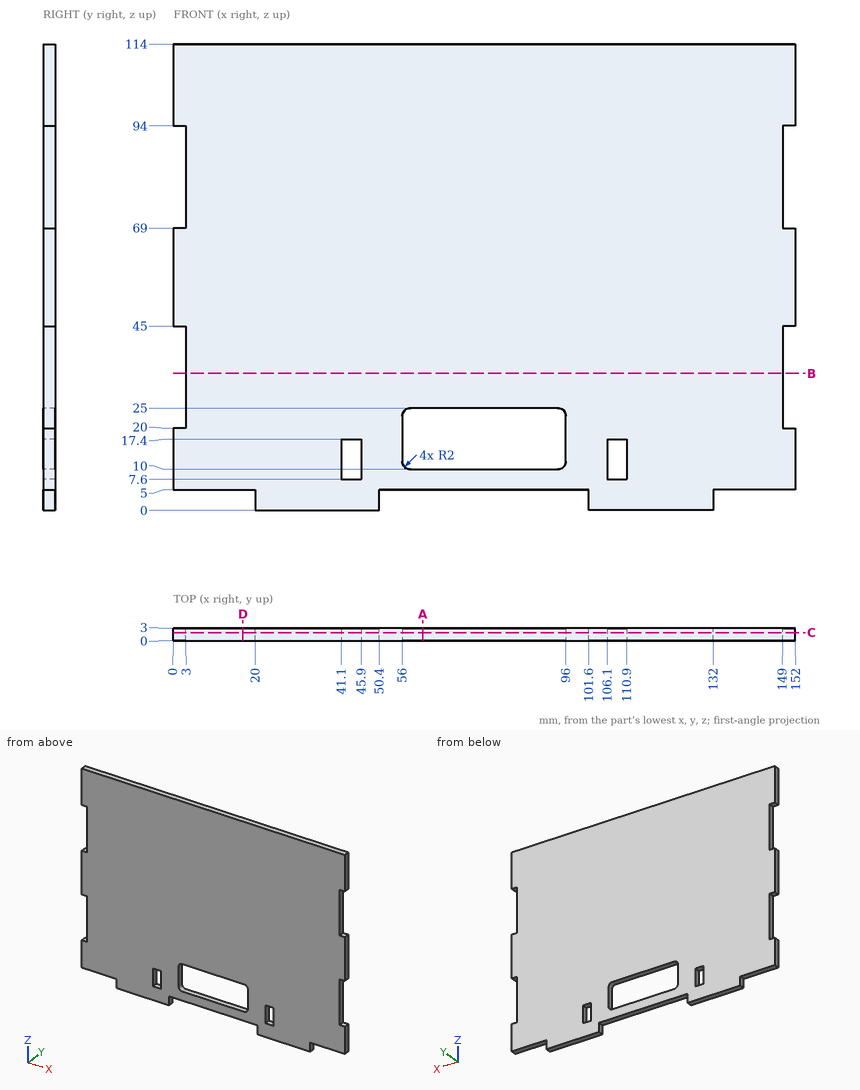
The drawing under review shows one solid part. Ordinate dimensions are in mm from its lowest x, y, z. Round coordinates to 2 decimals unless told otherwise and drop trailing zeros. Loops run counter-clockwise (first coordinate to the right, second up) from the corner with the lowest first, then second, coordinate; pieces in that order, holes last. Notation, with made-up numbers: (34, -35.5) - (76, -35.5) arc R25 ccw to (76, -1.5) - close; hole circle Ø9 at (62, 27.5). An arc over 180 degrees is marked (long way). Put each result on its own line as item: value. Start each with the question number.
1. For probe 1 along X at (y, z) = (1.05, 14.5); probe 2 along Z at (x, y) = (107, 1.8); probe 3 along Z at (x, y) = (62.5, 1.6), list the stretches that pass through material, from the lowest coordinate up. Write a range as [from, to].
2. Consider section B-B on z = 33.5. State the section outline as (x, y) points, plus the area to 3 significant figures.
3. Consider section A-A on x = 61. State the section outline as (y, z) points, plus the area to 3 significant figures.
4. Consider section C-C on y = 1.95. State how many separate pieces and enclosed holes the cut face has, plus the area to 3 significant figures.
5. Consider section D-D on x = 17. State the section outline as (y, z) points, plus the area to 3 significant figures.
6. Insertion check: P1, Ø0.9, axis at x = 13, y = 1, coming from the -Z side; P2, Ø0.9, axis at y = 2, z = 3.5, coming from the -X side; P3, Ø0.9, axis at y = 1, z = 3, coming from the +X side. Each pin has a flat end and moves straight along its axis. Give the tip position at first contact, or say it passes through.
Result sheet:
1. probe 1: [0, 41.1], [45.9, 56], [96, 106.1], [110.9, 152]
1. probe 2: [0, 7.6], [17.4, 114]
1. probe 3: [5, 10], [25, 114]
2. outline: (3, 0) - (149, 0) - (149, 3) - (3, 3) - close
2. area: 438 mm^2
3. outline: (0, 5) - (3, 5) - (3, 10) - (0, 10) - close; (0, 25) - (3, 25) - (3, 114) - (0, 114) - close
3. area: 282 mm^2
4. separate pieces: 1
4. enclosed holes: 3
4. area: 15,900 mm^2
5. outline: (0, 5) - (3, 5) - (3, 114) - (0, 114) - close
5. area: 327 mm^2
6. P1: z = 5
6. P2: x = 20
6. P3: x = 132
